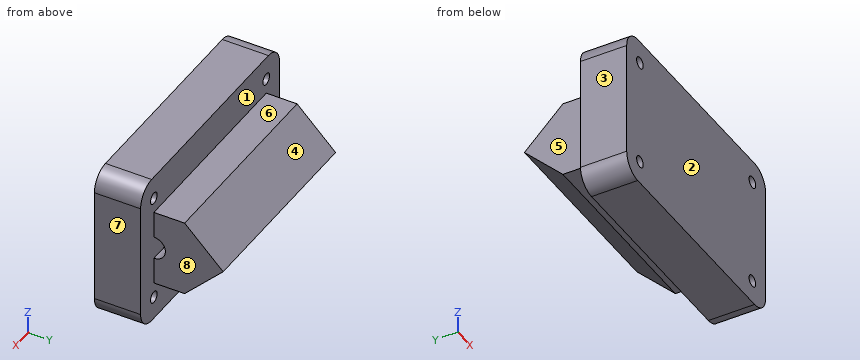
```python
from build123d import *

# Parameters (mm, degrees)
IZIM1_W                     = 315
IZIM1_H                     = 200
Y_KSEKLIK_EKSTR_ZYON1_DEPTH = 60
RADYUS1_R                   = 25
IZIM2_R                     = 7.5
KES_EKSTR_ZYON1_DEPTH       = 61
IZIM3_W                     = 255
IZIM3_H                     = 100
Y_KSEKLIK_EKSTR_ZYON2_DEPTH = 40
Y_KSEKLIK_EKSTR_ZYON3_DEPTH = 255
KES_EKSTR_ZYON2_DEPTH       = 286


with BuildPart() as part:
    # Çizim1 → Yükseklik-Ekstrüzyon1 (new body)
    with BuildSketch(Plane(origin=(0, 0, 0), x_dir=(1, 0, 0), z_dir=(0, 1, 0))):
        Rectangle(IZIM1_W, IZIM1_H)
    extrude(amount=Y_KSEKLIK_EKSTR_ZYON1_DEPTH)

    # Radyus1
    radyus1_edges = [part.edges().sort_by_distance(p)[0] for p in [
        (157.5, 30, 100),
        (-157.5, 30, 100),
        (-157.5, 30, -100),
        (157.5, 30, -100),
    ]]
    fillet(radyus1_edges, radius=RADYUS1_R)

    # Çizim2 → Kes-Ekstrüzyon1 (cut, through all)
    with BuildSketch(Plane(origin=(0, 60, 0), x_dir=(1, 0, 0), z_dir=(0, 1, 0))):
        with Locations((-127.5, 70)):
            Circle(IZIM2_R)
        with Locations((127.5, 70)):
            Circle(IZIM2_R)
        with Locations((127.5, -70)):
            Circle(IZIM2_R)
        with Locations((-127.5, -70)):
            Circle(IZIM2_R)
    extrude(amount=-KES_EKSTR_ZYON1_DEPTH, mode=Mode.SUBTRACT)

    # Çizim3 → Yükseklik-Ekstrüzyon2 (add)
    with BuildSketch(Plane(origin=(0, 60, 0), x_dir=(1, 0, 0), z_dir=(0, 1, 0))):
        Rectangle(IZIM3_W, IZIM3_H)
    extrude(amount=Y_KSEKLIK_EKSTR_ZYON2_DEPTH)

    # Çizim4 → Yükseklik-Ekstrüzyon3 (add)
    with BuildSketch(Plane(origin=(127.5, 0, 0), x_dir=(0, 0, -1), z_dir=(1, 0, 0))):
        Polygon((-50, 100), (0, 150), (50, 100), align=None)
    extrude(amount=-Y_KSEKLIK_EKSTR_ZYON3_DEPTH)

    # Çizim5 → Kes-Ekstrüzyon2 (cut, through all)
    with BuildSketch(Plane(origin=(127.5, 0, 0), x_dir=(0, 0, -1), z_dir=(1, 0, 0))):
        with BuildLine():
            Line((-15, 60), (15, 60))
            ThreePointArc((15, 60), (0, 75), (-15, 60))
        make_face()
    extrude(amount=-KES_EKSTR_ZYON2_DEPTH, mode=Mode.SUBTRACT)


solid = part.part
```
Could you check a few things on this model? Use its own coordinates, in mm. Face numbers are marked on the shaded views. A direction names the side the tool comes from. Give positions to 0.01 mm unless a question says otherwise; leave off trailing zeros. Loops run counter-clockwise (first coordinate to the right, second up) from the corner with the lowest first, then second, coordinate; pieces in that order, holes last. Notation, with made-up numbers: (-7, -32) -> (45, -32) arc R8 cw to (45, -26) -> close; hole circle Ø4 at (-6, 40.25). An arc over 180 degrees is marked (long way). Put each result on its own line as item: value.
(1) Please list where these lines run through material, in increasing order: probe 1 along Z at (x, y) = (127.5, 19.5); probe 2 along X at (y, z) = (45.5, -70); probe 3 along X at (y, z) = (26, -67.5). Write a range as [from, to].
Computed:
probe 1: [-100, -77.5], [-62.5, 62.5], [77.5, 100]
probe 2: [-157.5, -135], [-120, 120], [135, 157.5]
probe 3: [-157.5, -134.57], [-120.43, 120.43], [134.57, 157.5]
(2) For the marked faces 5, 6, 7 and 8, which set-ups out of +Z, -Z, +X, -X, +Y, -Y let a thin tool reach every point of the face, with its end or its side?
Computed:
face 5: +Z, -Z, -X, +Y
face 6: +Z, +X, -X, +Y
face 7: +Z, -Z, +X, +Y, -Y
face 8: +Z, -Z, +X, +Y
(3) Imagine slicing it at C-C on z = 44. Write out the boundary of the cut face in (x, y).
Computed:
outline: (-157.5, 0) -> (157.5, 0) -> (157.5, 60) -> (127.5, 60) -> (127.5, 106) -> (-127.5, 106) -> (-127.5, 60) -> (-157.5, 60) -> close
(4) I'm going to push flat-ended pins straight in: pin 1 Ø2 at (y, z) = (80, 16.5) entering from -X; pin 2 Ø12 at (x, y) = (8.5, 89) entering from +Z; pin 3 Ø19.5 at (x, z) = (127.5, -70) entering from +Y; pin 4 Ø12 at (x, z) = (-127.5, 70) entering from +Y. Where does each tip first touch, or does it pass through?
Computed:
pin 1: x = -127.5
pin 2: z = 50
pin 3: y = 60
pin 4: through
(5) Imagine slicing it at D-D on y = 139.5. Write out the boundary of the cut face in (x, z), plus the area to 4 significant figures.
Computed:
outline: (-127.5, -10.5) -> (127.5, -10.5) -> (127.5, 10.5) -> (-127.5, 10.5) -> close
area: 5,355 mm^2
(6) Imagine slicing it at A-A on z = 70. Write out the boundary of the cut face in (x, y).
Computed:
outline: (-157.5, 0) -> (-135, 0) -> (-135, 60) -> (-157.5, 60) -> close; (-120, 0) -> (120, 0) -> (120, 60) -> (-120, 60) -> close; (135, 0) -> (157.5, 0) -> (157.5, 60) -> (135, 60) -> close
(7) Imagine slicing it at B-B on x = 53. Write out the boundary of the cut face in (y, z).
Computed:
outline: (0, -100) -> (60, -100) -> (60, -50) -> (100, -50) -> (150, 0) -> (100, 50) -> (60, 50) -> (60, 100) -> (0, 100) -> close; hole (60, -15) arc R15 ccw to (60, 15) -> close
(8) Thinking about a two-plate mould opening in Y: for the marked faces 1, 2, 3 and 4, which applies, pulls with the +Y half, pulls with the -Y half, needs draft (parallel to the pull), parting line crosses it, or undercut?
Computed:
face 1: undercut
face 2: pulls with the -Y half
face 3: needs draft
face 4: pulls with the +Y half
